Check sheet for the drawn part. Datum: minimum x, y, z corner. Units: mm. A direction names the side the tool comes from. Coordinates: 2 decimals unless noted, no trailing zeros. Order: outer loops, then holes, each group sorted by start corner. A loop starts at its lowest first (then second) coordinate and runs counter-clockwise, first axis right, second up.
1. Cross-section at A-A (x = 5). Enter the section's corners in (y, z), then the cut area to 3 significant figures.
2. Cross-section at D-D (y = 12). Enter the section's corners in (x, z), then the cut area to 3 significant figures.
3. Set-up check for the marked faces 1 and 2: record each of +Z, -Z, +X, -X, +Y, -Y from which the full face is reachable in a straight line by a thin tool's end or side.
4. Gauge pin test, flat end, axial feed: pin 1 Ø3 at (x, y) = (36, 8.5) entering from +Z. Record the tip position at first contact, or that the pin passes through.
5. Thickness scan on line 1 (X direction, y = 8, z = 8.95); line 2 (Y direction, x = 20, z = 4); line 3 (X direction, y = 8, z = 5). Record the ranges inside material, lowest first.
6. Cross-section at C-C (z = 10.75). Enter the section's corners in (x, y), then the cut area to 3 significant figures.
7. Cross-section at B-B (y = 8). Enter the section's corners in (x, z), then the cut area to 3 significant figures.
8. Draft check along X on the marked faces 3, 4, 5 and 6. Enter one of: released by +X, released by -X, zero draft, split by the parting line, or undercut.
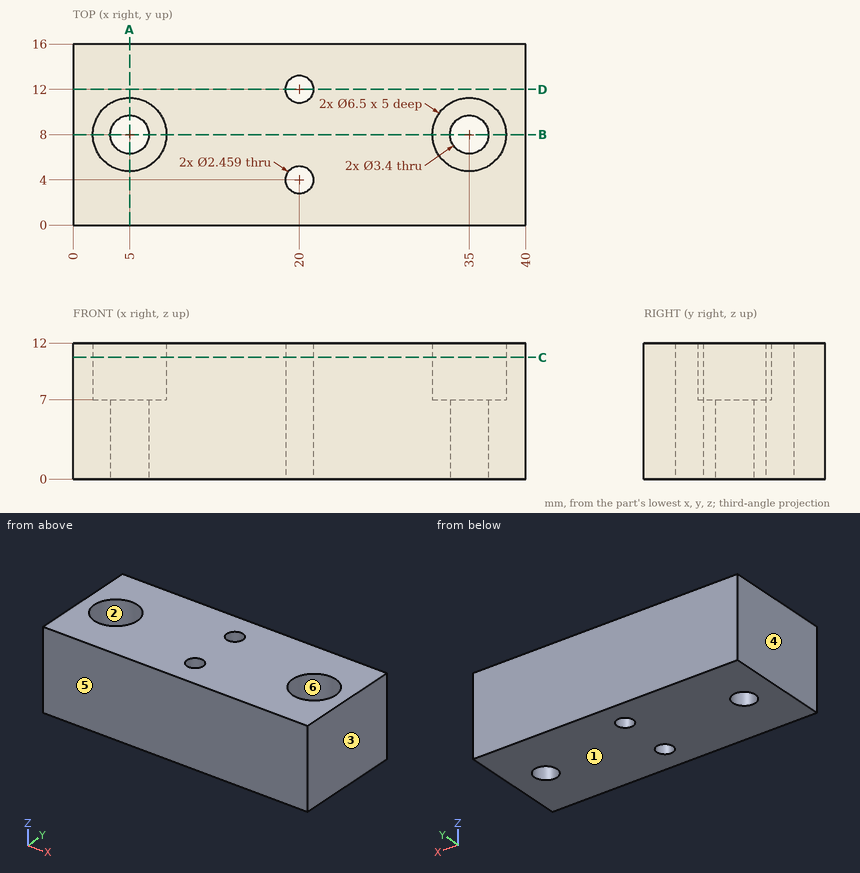
Data:
1. outline: (0, 0) - (6.3, 0) - (6.3, 7) - (4.75, 7) - (4.75, 12) - (0, 12) - close; (9.7, 0) - (16, 0) - (16, 12) - (11.25, 12) - (11.25, 7) - (9.7, 7) - close
1. area: 136 mm2
2. outline: (0, 0) - (18.77, 0) - (18.77, 12) - (0, 12) - close; (21.23, 0) - (40, 0) - (40, 12) - (21.23, 12) - close
2. area: 450 mm2
3. face 1: -Z, +X, -X, +Y, -Y
3. face 2: +Z
4. pin 1: stops at z = 7
5. line 1: x = 0 to 1.75, 8.25 to 31.75, 38.25 to 40
5. line 2: y = 0 to 2.77, 5.23 to 10.77, 13.23 to 16
5. line 3: x = 0 to 3.3, 6.7 to 33.3, 36.7 to 40
6. outline: (0, 0) - (40, 0) - (40, 16) - (0, 16) - close; hole circle Ø6.5 at (5, 8); hole circle Ø2.46 at (20, 4); hole circle Ø2.46 at (20, 12); hole circle Ø6.5 at (35, 8)
6. area: 564 mm2
7. outline: (0, 0) - (3.3, 0) - (3.3, 7) - (1.75, 7) - (1.75, 12) - (0, 12) - close; (6.7, 0) - (33.3, 0) - (33.3, 7) - (31.75, 7) - (31.75, 12) - (8.25, 12) - (8.25, 7) - (6.7, 7) - close; (36.7, 0) - (40, 0) - (40, 12) - (38.25, 12) - (38.25, 7) - (36.7, 7) - close
7. area: 367 mm2
8. face 3: released by +X
8. face 4: released by -X
8. face 5: zero draft
8. face 6: undercut
